Can you work these out from the model? Positions are in its coordinate system, mm. Give positions to 0.01 mm unless a question says otherwise; leave off trailing zeros. Order: outer loops, then holes, each group sorted by start corner. A loop starts at its lowest first (then second) coordinate and runs counter-clockwise, first axis right, second up. Notation, with made-up numbers: (30.25, 30) -> (68.25, 30) arc R27 ccw to (68.25, 51) -> close; hole circle Ø6 at (1, 85.25). An arc over 180 degrees is marked (long way). Answer as CSV lines item,"result".
```python
from build123d import *

# Parameters (mm, degrees)
CYLINDER1669_R     = 2.5
CYLINDER1669_DEPTH = 20
CYLINDER1668_R     = 2.5
CYLINDER1668_DEPTH = 20
CYLINDER1667_R     = 5
CYLINDER1667_DEPTH = 5
CYLINDER1666_R     = 5
CYLINDER1666_DEPTH = 5
CYLINDER1647_R     = 1.5
CYLINDER1647_DEPTH = 60
CYLINDER1648_R     = 1.5
CYLINDER1648_DEPTH = 60
CYLINDER1649_R     = 1.5
CYLINDER1649_DEPTH = 60
CYLINDER1646_R     = 1.5
CYLINDER1646_DEPTH = 60
CYLINDER1619_R     = 3
CYLINDER1619_DEPTH = 48
BOX644_W           = 90
BOX644_H           = 20
BOX644_DEPTH       = 4
CHAMFER042_SIZE    = 4
CHAMFER043_SIZE    = 2


with BuildPart() as obj1:
    # Cylinder1669 → Cylinder1669 (new body)
    with BuildSketch(Plane(origin=(-35, 90, -59), x_dir=(1, 0, 0), z_dir=(0, 0, 1))):
        Circle(CYLINDER1669_R)
    extrude(amount=CYLINDER1669_DEPTH)


with BuildPart() as compound819:
    # Cylinder1668 → Cylinder1668 (new body)
    with BuildSketch(Plane(origin=(35, 90, -59), x_dir=(1, 0, 0), z_dir=(0, 0, 1))):
        Circle(CYLINDER1668_R)
    extrude(amount=CYLINDER1668_DEPTH)

    # Compound819: union obj1
    add(obj1.part)


with BuildPart() as compound819_1:
    # Compound819 placement: moved
    add(compound819.part.moved(Location((0, 0, 18))))


with BuildPart() as obj2:
    # Cylinder1667 → Cylinder1667 (new body)
    with BuildSketch(Plane(origin=(-35, 90, -59), x_dir=(1, 0, 0), z_dir=(0, 0, 1))):
        Circle(CYLINDER1667_R)
    extrude(amount=CYLINDER1667_DEPTH)


with BuildPart() as compound818:
    # Cylinder1666 → Cylinder1666 (new body)
    with BuildSketch(Plane(origin=(35, 90, -59), x_dir=(1, 0, 0), z_dir=(0, 0, 1))):
        Circle(CYLINDER1666_R)
    extrude(amount=CYLINDER1666_DEPTH)

    # Compound818: union obj2
    add(obj2.part)


with BuildPart() as compound818_1:
    # Compound818 placement: moved
    add(compound818.part.moved(Location((0, 0, 29))))


with BuildPart() as obj3:
    # Cylinder1647 → Cylinder1647 (new body)
    with BuildSketch(Plane(origin=(18, 85, -57), x_dir=(1, 0, 0), z_dir=(0, 0, 1))):
        Circle(CYLINDER1647_R)
    extrude(amount=CYLINDER1647_DEPTH)


with BuildPart() as obj4:
    # Cylinder1648 → Cylinder1648 (new body)
    with BuildSketch(Plane(origin=(-18, 85, -57), x_dir=(1, 0, 0), z_dir=(0, 0, 1))):
        Circle(CYLINDER1648_R)
    extrude(amount=CYLINDER1648_DEPTH)


with BuildPart() as obj5:
    # Cylinder1649 → Cylinder1649 (new body)
    with BuildSketch(Plane(origin=(-18, 95, -57), x_dir=(1, 0, 0), z_dir=(0, 0, 1))):
        Circle(CYLINDER1649_R)
    extrude(amount=CYLINDER1649_DEPTH)


with BuildPart() as compound812:
    # Cylinder1646 → Cylinder1646 (new body)
    with BuildSketch(Plane(origin=(18, 95, -57), x_dir=(1, 0, 0), z_dir=(0, 0, 1))):
        Circle(CYLINDER1646_R)
    extrude(amount=CYLINDER1646_DEPTH)

    # Compound812: union obj3, obj4, obj5
    add(obj3.part)
    add(obj4.part)
    add(obj5.part)


with BuildPart() as obj6:
    # Cylinder1619 → Cylinder1619 (new body)
    with BuildSketch(Plane(origin=(0, 90, -55), x_dir=(1, 0, 0), z_dir=(0, 0, 1))):
        Circle(CYLINDER1619_R)
    extrude(amount=CYLINDER1619_DEPTH)


with BuildPart() as chamfer043:
    # Box644 → Box644 (new body)
    with BuildSketch(Plane(origin=(-45, 80, -32), x_dir=(1, 0, 0), z_dir=(0, 0, 1))):
        with Locations((45, 10)):
            Rectangle(BOX644_W, BOX644_H)
    extrude(amount=BOX644_DEPTH)

    # Cut313: cut obj6
    add(obj6.part, mode=Mode.SUBTRACT)

    # Cut324: cut Compound812
    add(compound812.part, mode=Mode.SUBTRACT)

    # Cut331: cut Compound818
    add(compound818_1.part, mode=Mode.SUBTRACT)

    # Cut332: cut Compound819
    add(compound819_1.part, mode=Mode.SUBTRACT)

    # Chamfer042
    chamfer042_edges = [chamfer043.edges().sort_by_distance(p)[0] for p in [
        (-45, 100, -30),
        (45, 100, -30),
    ]]
    chamfer(chamfer042_edges, length=CHAMFER042_SIZE)

    # Chamfer043
    chamfer043_edges = [chamfer043.edges().sort_by_distance(p)[0] for p in [
        (-45, 88, -28),
        (45, 88, -28),
    ]]
    chamfer(chamfer043_edges, length=CHAMFER043_SIZE)


solid = chamfer043.part
```
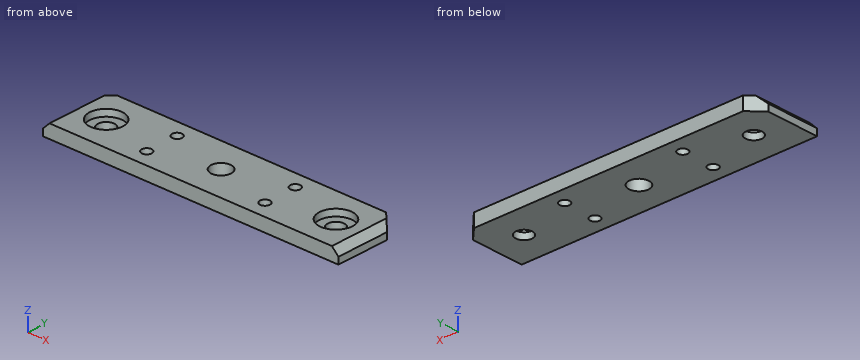
Item 1: Please list where these lines run through material, in increasing order: line 1 along X through (y, z) = (85, -30.3); line 2 along Y through (x, z) = (-18, -29.25); line 3 along Y through (x, z) = (-35, -28.6).
Numbers:
line 1,"x = -45 to -19.5, -16.5 to 16.5, 19.5 to 45"
line 2,"y = 80 to 83.5, 86.5 to 93.5, 96.5 to 100"
line 3,"y = 80 to 85, 95 to 100"
Item 2: For pin 1 (5 mm diameter, centred on x = 35, y = 90.5, fed in from +Z), with a flat end and sliding along its axis, tell me the tip position at first contact or that it passes through.
Numbers:
pin 1,"stops at z = -30"
Item 3: Imagine slicing it at C-C, the plane z = -29.25. Please give me the cut outline in (x, y).
Numbers:
outline,"(-44.25, 80) -> (44.25, 80) -> (44.25, 96.75) -> (41, 100) -> (-41, 100) -> (-44.25, 96.75) -> close; hole circle Ø10 at (-35, 90); hole circle Ø3 at (-18, 85); hole circle Ø3 at (-18, 95); hole circle Ø6 at (0, 90); hole circle Ø3 at (18, 85); hole circle Ø3 at (18, 95); hole circle Ø10 at (35, 90)"
Item 4: Imagine slicing it at A-A, the plane x = -18. Please give me the cut outline in (y, z).
Numbers:
outline,"(80, -32) -> (83.5, -32) -> (83.5, -28) -> (80, -28) -> close; (86.5, -32) -> (93.5, -32) -> (93.5, -28) -> (86.5, -28) -> close; (96.5, -32) -> (100, -32) -> (100, -28) -> (96.5, -28) -> close"
Item 5: Imagine slicing it at D-D, the plane x = 35. Please give me the cut outline in (y, z), then the cut area to 3 significant figures.
Numbers:
outline,"(80, -32) -> (87.5, -32) -> (87.5, -30) -> (85, -30) -> (85, -28) -> (80, -28) -> close; (92.5, -32) -> (100, -32) -> (100, -28) -> (95, -28) -> (95, -30) -> (92.5, -30) -> close"
area,"50.0 mm²"
Item 6: Imagine slicing it at B-B, the plane y = 90. Please give me the cut outline in (x, z).
Numbers:
outline,"(-45, -32) -> (-37.5, -32) -> (-37.5, -30) -> (-40, -30) -> (-40, -28) -> (-43, -28) -> (-45, -30) -> close; (-32.5, -32) -> (-3, -32) -> (-3, -28) -> (-30, -28) -> (-30, -30) -> (-32.5, -30) -> close; (3, -32) -> (32.5, -32) -> (32.5, -30) -> (30, -30) -> (30, -28) -> (3, -28) -> close; (37.5, -32) -> (45, -32) -> (45, -30) -> (43, -28) -> (40, -28) -> (40, -30) -> (37.5, -30) -> close"
